Here's how the part is built. I have some questions about the finished solid (model axes, mm). Round coordinates to 2 decimals unless told otherwise and drop trailing zeros. Write each loop counter-clockwise with the first axis right and the second up, starting at its lowest first coordinate (ties: lowest second). Pieces come first, ordered by that corner, then holes. Notation, with made-up numbers: (7, 57) -> (66, 57) arc R27 ccw to (66, 85) -> close; hole circle Ø6 at (7, 33). An arc over 180 degrees is marked (long way). Answer in a Markdown table with one row per item.
from build123d import *

# Parameters (mm, degrees)
F0_R     = 2.5527
F1_DEPTH = 3.175


# Not quite as in the source:
# - a length typed as a fraction of an inch, garbled in the dataset ("3 / 203.2 mm" for 3/8 in), is restored


with BuildPart() as f1:
    # F0 (on Top) → F1 (new body)
    with BuildSketch(Plane.XY):
        Polygon((0, 25.4), (0, 0), (101.6, 0), (101.6, 101.6), (76.2, 101.6), (76.2, 25.4), align=None)
        with Locations((12.7, 12.7)):
            Circle(F0_R, mode=Mode.SUBTRACT)
        with Locations((25.4, 12.7)):
            Circle(F0_R, mode=Mode.SUBTRACT)
        with Locations((38.1, 12.7)):
            Circle(F0_R, mode=Mode.SUBTRACT)
        with Locations((50.8, 12.7)):
            Circle(F0_R, mode=Mode.SUBTRACT)
        with Locations((63.5, 12.7)):
            Circle(F0_R, mode=Mode.SUBTRACT)
        with Locations((76.2, 12.7)):
            Circle(F0_R, mode=Mode.SUBTRACT)
        with Locations((88.9, 12.7)):
            Circle(F0_R, mode=Mode.SUBTRACT)
        with Locations((88.9, 25.4)):
            Circle(F0_R, mode=Mode.SUBTRACT)
        with Locations((88.9, 38.1)):
            Circle(F0_R, mode=Mode.SUBTRACT)
        with Locations((88.9, 50.8)):
            Circle(F0_R, mode=Mode.SUBTRACT)
        with Locations((88.9, 63.5)):
            Circle(F0_R, mode=Mode.SUBTRACT)
        with Locations((88.9, 76.2)):
            Circle(F0_R, mode=Mode.SUBTRACT)
        with Locations((88.9, 88.9)):
            Circle(F0_R, mode=Mode.SUBTRACT)
        Polygon((76.2, 101.6), (0, 25.4), (76.2, 25.4), align=None)
    extrude(amount=F1_DEPTH)


solid = f1.part
1) We'd pull the mould along Y, two halves only. Please class faces 1 (the face through (50, 0, 2)), 2 (the face through (0, 13, 2)), 3 (the face through (90.078, 86.635, 1.565)): +Y half, -Y half, draft (parallel to the pull), parting line (faces both ways), or undercut.
Response:
| item | result |
|---|---|
| face 1 | -Y half |
| face 2 | draft |
| face 3 | undercut |
2) I want a section at A-A, the plane x = 88.9. Count the separate pieces of the cut face and the enclosed holes in it, and give its area (3 significant figures).
Response:
| item | result |
|---|---|
| separate pieces | 8 |
| enclosed holes | 0 |
| area | 209 mm^2 |
3) For pin 1 (6.5 mm diameter, centred on x = 25.4, y = 12.7, fed in from +Z) (3 decimals), with a flat end and sliding along its axis, tell me the tip position at first contact or that it passes through.
Response:
| item | result |
|---|---|
| pin 1 | stops at z = 3.175 |
4) I want a section at B-B, the plane y = 76.2. List the corners of the cut face in (x, z) for me (3 decimals).
Response:
| item | result |
|---|---|
| outline | (50.8, 0) -> (86.347, 0) -> (86.347, 3.175) -> (50.8, 3.175) -> close; (91.453, 0) -> (101.6, 0) -> (101.6, 3.175) -> (91.453, 3.175) -> close |
5) I want a section at C-C, the plane x = 38.1. List the corners of the cut face in (y, z) for me (3 decimals).
Response:
| item | result |
|---|---|
| outline | (0, 0) -> (10.147, 0) -> (10.147, 3.175) -> (0, 3.175) -> close; (15.253, 0) -> (63.5, 0) -> (63.5, 3.175) -> (15.253, 3.175) -> close |
6) I need wall thicknesses on line 1 (Y direction, x = 76.2, z = 2.2); line 2 (Y direction, x = 64, z = 0.8); line 3 (X direction, y = 62, z = 3.05). Which ranges of each line are inside material? Lowest first, please. Write a range as [from, to].
Response:
| item | result |
|---|---|
| line 1 | y = [0, 10.15], [15.25, 101.6] |
| line 2 | y = [0, 10.2], [15.2, 89.4] |
| line 3 | x = [36.6, 86.83], [90.97, 101.6] |
